```python
from build123d import *

# Parameters (mm, degrees)
F1_DEPTH = 25


with BuildPart() as f1:
    # F0 (on Top) → F1 (new body)
    with BuildSketch(Plane.XY):
        with BuildLine():
            Line((32.09034, 33.209568), (32.09034, 48.417067))
            Line((32.09034, 48.417067), (-34.191456, 48.417067))
            Line((-34.191456, 48.417067), (-34.191667, 23.417067))
            Line((-34.191667, 23.417067), (-54.191667, 23.417236))
            Line((-54.191667, 23.417236), (-54.19166, -23.416399))
            Line((-54.19166, -23.416399), (-34.19166, -23.416568))
            Line((-34.19166, -23.416568), (-34.19166, -48.416568))
            Line((-34.19166, -48.416568), (32.09034, -48.416568))
            Line((32.09034, -48.416568), (32.09034, -33.209568))
            ThreePointArc((32.09034, -33.209568), (-11.042779, 0), (32.09034, 33.209568))
        make_face()
    extrude(amount=F1_DEPTH)


solid = f1.part
```
Could you check a few things on this model? Use its own coordinates, in mm. A direction names the side the tool comes from. Round coordinates to 2 decimals unless told otherwise and drop trailing zeros. Loops run counter-clockwise (first coordinate to the right, second up) from the corner with the lowest first, then second, coordinate; pieces in that order, holes last. Notation, with made-up numbers: (29, -4.5) -> (52, -4.5) arc R32 ccw to (52, 32.5) -> close; hole circle Ø3 at (31.5, 24). An arc over 180 degrees is marked (long way). Put each result on its own line as item: value.
Q1. I want a section at D-D on y = 13. Write out the boundary of the cut face in (x, z), and give its area (3 significant figures).
Checks:
outline: (-54.19, 0) -> (-8.49, 0) -> (-8.49, 25) -> (-54.19, 25) -> close
area: 1,140 mm2
Q2. For pin 1 Ø10 at (x, z) = (-41, 17) entering from -Y; pin 2 Ø12.5 at (y, z) = (-36, 15) entering from -X; pin 3 Ø6 at (x, z) = (-49, 15) entering from +Y, each with a flat end and sliding along its axis, tell me the tip position at first contact or that it passes through.
Checks:
pin 1: y = -23.42
pin 2: x = -34.19
pin 3: y = 23.42
Q3. I want a section at C-C on y = 0. Write out the boundary of the cut face in (x, z), and give its area (3 significant figures).
Checks:
outline: (-54.19, 0) -> (-11.04, 0) -> (-11.04, 25) -> (-54.19, 25) -> close
area: 1,080 mm2
Q4. Please list where these lines run through material, in increasing order: line 1 (X direction, y = 0, z = 9); line 2 (Y direction, x = -41, z = 3.5); line 3 (X direction, y = -34.5, z = 7). Write a range as from..to.
Checks:
line 1: -54.19..-11.04
line 2: -23.42..23.42
line 3: -34.19..32.09
Q5. I want a section at A-A on x = 1. Write out the boundary of the cut face in (y, z).
Checks:
outline: (-48.42, 0) -> (-26.12, 0) -> (-26.12, 25) -> (-48.42, 25) -> close; (26.12, 0) -> (48.42, 0) -> (48.42, 25) -> (26.12, 25) -> close
Q6. Thinking about a two-plate mould opening in Y: for faces 3 (the flat face through (-2, -48.417, 12)), 4 (the flat face through (-1, 48.417, 12)), 5 (the flat face through (-54.192, 0, 12)), 6 (the cylindrical face through (-11.03, -0.88, 12.32)), which applies, pulls with the +Y half, pulls with the -Y half, needs draft (parallel to the pull), parting line crosses it, or undercut?
Checks:
face 3: pulls with the -Y half
face 4: pulls with the +Y half
face 5: needs draft
face 6: undercut
Q7. Which directions (+Z, -Z, +X, -X, +Y, -Y) give clear straight access to the entire face, cutting with the end or side of a thin tool? Please do faces 1 (the flat face through (-21, 1, 0)), 2 (the flat face through (-34.192, -36, 12)).
Checks:
face 1: -Z, +X, -X, +Y, -Y
face 2: +Z, -Z, -X, -Y
Q8. I want a section at B-B on z = 21. Write out the boundary of the cut face in (x, y).
Checks:
outline: (-54.19, -23.42) -> (-34.19, -23.42) -> (-34.19, -48.42) -> (32.09, -48.42) -> (32.09, -33.21) arc R34.35 cw (long way) to (32.09, 33.21) -> (32.09, 48.42) -> (-34.19, 48.42) -> (-34.19, 23.42) -> (-54.19, 23.42) -> close
